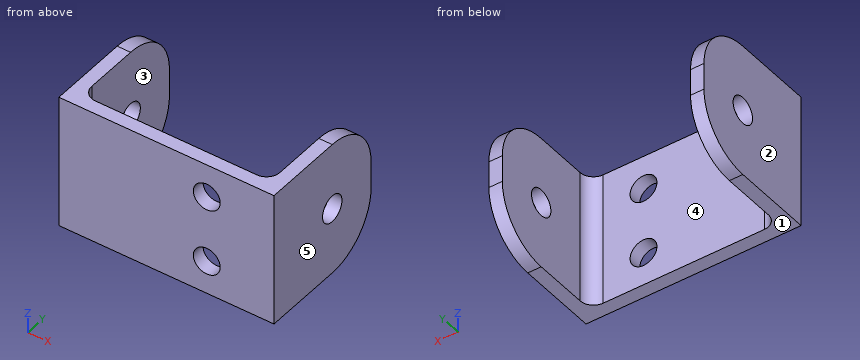
from build123d import *

# Parameters (mm, degrees)
SKETCH1_W           = 50.8
SKETCH1_H           = 31.75
BOSS_EXTRUDE1_DEPTH = 15.875
SKETCH2_W           = 44.45
SKETCH2_H           = 28.575
CUT_EXTRUDE1_DEPTH  = 32.75
SKETCH3_R           = 3.175
CUT_EXTRUDE2_DEPTH  = 4.175
FILLET1_R           = 3.175
SKETCH4_R           = 3.175
CUT_EXTRUDE3_DEPTH  = 51.8
FILLET2_R           = 12.7


with BuildPart() as part:
    # Sketch1 → Boss-Extrude1 (new body, symmetric)
    with BuildSketch(Plane.XY):
        Rectangle(SKETCH1_W, SKETCH1_H)
    extrude(amount=BOSS_EXTRUDE1_DEPTH, both=True)

    # Sketch2 → Cut-Extrude1 (cut, through all)
    with BuildSketch(Plane.XY.offset(15.875)):
        with Locations((0, 1.5875)):
            Rectangle(SKETCH2_W, SKETCH2_H)
    extrude(amount=-CUT_EXTRUDE1_DEPTH, mode=Mode.SUBTRACT)

    # Sketch3 → Cut-Extrude2 (cut, through all)
    with BuildSketch(Plane(origin=(0, -12.7, 0), x_dir=(1, 0, 0), z_dir=(0, 1, 0))):
        with Locations((9.525, 7.9375)):
            Circle(SKETCH3_R)
        with Locations((9.525, -7.9375)):
            Circle(SKETCH3_R)
    extrude(amount=-CUT_EXTRUDE2_DEPTH, mode=Mode.SUBTRACT)

    # Fillet1
    fillet1_edges = [part.edges().sort_by_distance(p)[0] for p in [
        (-22.225, -12.7, 0),
        (22.225, -12.7, 0),
    ]]
    fillet(fillet1_edges, radius=FILLET1_R)

    # Sketch4 → Cut-Extrude3 (cut, through all)
    with BuildSketch(Plane(origin=(25.4, 0, 0), x_dir=(0, 0, -1), z_dir=(1, 0, 0))):
        with Locations((0, 3.175)):
            Circle(SKETCH4_R)
    extrude(amount=-CUT_EXTRUDE3_DEPTH, mode=Mode.SUBTRACT)

    # Fillet2
    fillet2_edges = [part.edges().sort_by_distance(p)[0] for p in [
        (-23.8125, 15.875, -15.875),
        (-23.8125, 15.875, 15.875),
        (23.8125, 15.875, -15.875),
        (23.8125, 15.875, 15.875),
    ]]
    fillet(fillet2_edges, radius=FILLET2_R)


solid = part.part
Geometry check sheet. Reference: the model listing, model coordinates, mm. Face numbers are marked on the shaded views. A direction names the side the tool comes from. Round coordinates to 2 decimals unless told otherwise and drop trailing zeros. Order: outer loops, then holes, each group sorted by start corner. A loop starts at its lowest first (then second) coordinate and runs counter-clockwise, first axis right, second up. Notation, with made-up numbers: M 86,-34.5 L 121,-34.5 A27 ccw 121,-3.5 Z; hole C 30.25,52 d8. An arc over 180 degrees is marked long. Answer in a Markdown table with one row per item. Add a question column.
Item 1: Set-up check for the marked faces 4 and 5: record each of +Z, -Z, +X, -X, +Y, -Y from which the full face is reachable in a straight line by a thin tool's end or side.
Item 2: Depth check by flat-ended pin: pin 1 Ø6 at (x, z) = (-7, -2.5) entering from +Y; pin 2 Ø8 at (x, z) = (18.5, 12) entering from +Y. Enter the tip coordinate at first touch or a pass-through.
Item 3: Material ranges on L1, parallel to X at y = -5.5, z = -12.5 (3 decimals); L2, parallel to Y at x = 23, z = 0 (3 decimals); L3, parallel to Y at x = -8, z = -8.5 (3 decimals), recorded low to high. Write a range as [from, to].
Item 4: Draft check along X on the marked faces 1, 2 and 3. Enter one of: released by +X, released by -X, zero draft, split by the parting line, or undercut.
Item 5: Sectioned sample at A-A, the plane z = 0. Enter the section's corners in (x, y) (3 decimals).
Item 6: Sectioned sample at B-B, the plane y = -2. Enter the section's corners in (x, z) (3 decimals), plus the area to 3 significant figures.
Item 7: Sectioned sample at D-D, the plane x = 8. Enter the section's corners in (y, z) (3 decimals), plus the area to 3 significant figures.
Filled in:
| question | item | result |
|---|---|---|
| 1 | face 4 | +Z, -Z, +Y |
| 1 | face 5 | +Z, -Z, +X, +Y, -Y |
| 2 | pin 1 | stops at y = -12.7 |
| 2 | pin 2 | stops at y = 13.52 |
| 3 | L1 | x = [-25.4, -22.225], [22.225, 25.4] |
| 3 | L2 | y = [-15.875, 0], [6.35, 15.875] |
| 3 | L3 | y = [-15.875, -12.7] |
| 4 | face 1 | zero draft |
| 4 | face 2 | released by -X |
| 4 | face 3 | undercut |
| 5 | outline | M -25.4,-15.875 L 25.4,-15.875 L 25.4,0 L 22.225,0 L 22.225,-9.525 A3.175 cw 19.05,-12.7 L -19.05,-12.7 A3.175 cw -22.225,-9.525 L -22.225,0 L -25.4,0 Z; M -25.4,6.35 L -22.225,6.35 L -22.225,15.875 L -25.4,15.875 Z; M 22.225,6.35 L 25.4,6.35 L 25.4,15.875 L 22.225,15.875 Z |
| 6 | outline | M -25.4,-15.875 L -22.225,-15.875 L -22.225,15.875 L -25.4,15.875 Z; M 22.225,-15.875 L 25.4,-15.875 L 25.4,15.875 L 22.225,15.875 Z |
| 6 | area | 202 mm² |
| 7 | outline | M -15.875,-15.875 L -12.7,-15.875 L -12.7,-10.722 L -15.875,-10.722 Z; M -15.875,-5.153 L -12.7,-5.153 L -12.7,5.153 L -15.875,5.153 Z; M -15.875,10.722 L -12.7,10.722 L -12.7,15.875 L -15.875,15.875 Z |
| 7 | area | 65.4 mm² |
